Read the model definition and answer for the solid it produces. Units are mm, in the model's axes. Coordinates: 2 decimals unless noted, no trailing zeros. Order: outer loops, then holes, each group sorted by start corner. A loop starts at its lowest first (then second) coordinate and runs counter-clockwise, first axis right, second up. Notation, with made-up numbers: (15, -32.75) - (64, -32.75) arc R15 ccw to (64, -25.75) - close; hole circle Ø7 at (85.25, 60.5). An arc over 180 degrees is marked (long way). Use one line per item in the form item = value.
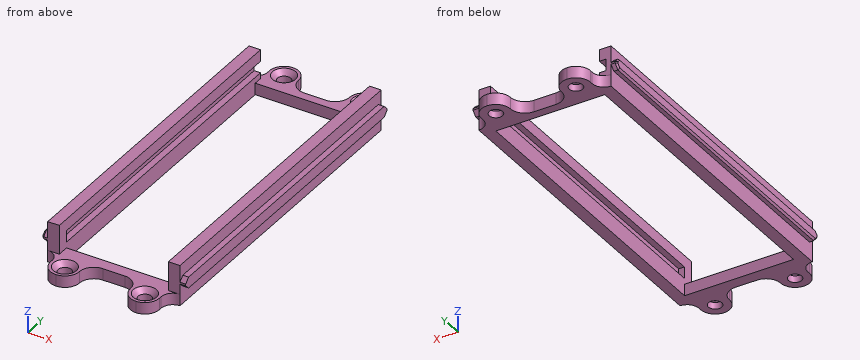
Autodesk Fusion 360 part; units mm, degrees
sketch "Sketch1" plane through (0, 0, 0) normal (1, 0, 0) x (0, 1, 0)
  line L0 (0, 0) -> (56.1898, 0)
  line L1 (56.1898, 0) -> (56.1898, 7)
  line L2 (56.1898, 7) -> (0, 7)
  line L3 (0, 7) -> (0, 0)
  dimension "d1" = 7
extrude "Extrude1" add sketch "Sketch1" along normal blind 1
sketch "Sketch2" plane through (1, 0, 0) normal (1, 0, 0) x (0, 1, 0)
  line L0 (0, 7) -> (0, 0)
  line L1 (0, 0) -> (56.1898, 0)
  line L2 (56.1898, 0) -> (56.1898, 7)
  line L3 (56.1898, 7) -> (0, 7)
  line L4 (0, 0) -> (56.1898, 0)
  line L5 (56.1898, 0) -> (56.1898, 3)
  line L6 (56.1898, 3) -> (0, 3)
  line L7 (0, 3) -> (0, 0)
  line L8 (0, 7) -> (56.1898, 7)
  line L9 (56.1898, 7) -> (56.1898, 5)
  line L10 (56.1898, 5) -> (0, 5)
  line L11 (0, 5) -> (0, 7)
  line L12 (0, 3) -> (2, 3)
  line L13 (2, 3) -> (2, 5)
  line L14 (2, 5) -> (0, 5)
  line L15 (0, 5) -> (0, 3)
  dimension "d4" = 3
  dimension "d5" = 2
  dimension "d12" = 2
extrude "Extrude2" add sketch "Sketch2" along normal blind 1 contours L0 L2 L3 L8 L9 L10 L11 L14 | L0 L6 L10 L12 L13 L14 L15 | L0 L1 L2 L4 L5 L6 L7 L12
sketch "Sketch3" plane through (0, 0, 0) normal (-1, 0, 0) x (0, -1, 0)
  line L0 (0, 0) -> (0, 7)
  line L1 (0, 7) -> (-56.1898, 7)
  line L2 (-56.1898, 7) -> (-56.1898, 0)
  line L3 (-56.1898, 0) -> (0, 0)
  line L4 (-56.1898, 3) -> (0, 3)
  line L5 (0, 3) -> (0, 4.9)
  line L6 (0, 4.9) -> (-56.1898, 4.9)
  line L7 (-56.1898, 4.9) -> (-56.1898, 3)
  dimension "d8" = 1.9
  dimension "d9" = 3
extrude "Extrude3" add sketch "Sketch3" along normal blind 1 contours L0 L2 L4 L5 L6 L7
sketch "Sketch4" plane through (2, 0, 0) normal (1, 0, 0) x (0, 1, 0)
  line L0 (0, 7) -> (0, 0)
  line L1 (0, 0) -> (56.1898, 0)
  line L2 (56.1898, 0) -> (56.1898, 3)
  line L3 (56.1898, 3) -> (2, 3)
  line L4 (2, 3) -> (2, 5)
  line L5 (2, 5) -> (56.1898, 5)
  line L6 (56.1898, 5) -> (56.1898, 7)
  line L7 (56.1898, 7) -> (0, 7)
  line L8 (0, 0) -> (2, 0)
  line L9 (2, 0) -> (2, 2)
  line L10 (2, 2) -> (0, 2)
  line L11 (0, 2) -> (0, 0)
  line L12 (56.1898, 0) -> (54.6898, 0)
  line L13 (54.6898, 0) -> (54.6898, 2)
  line L14 (54.6898, 2) -> (56.1898, 2)
  line L15 (56.1898, 2) -> (56.1898, 0)
  dimension "d13" = 2
  dimension "d14" = 2
  dimension "d15" = 1.5
  dimension "d16" = 2
extrude "Extrude4" add sketch "Sketch4" along normal blind 9.4 contours L0 L1 L8 L9 L10 L11 | L1 L2 L12 L13 L14 L15
mirror "Mirror1" about plane through (11.4, 0, 0) normal (1, 0, 0) of bodies 1 merged
extrude "Extrude5" cut 1 faces at (1, 20.0633, 4.3333) along direction (1, 0, 0) blind 0.1
extrude "Extrude6" cut 1 faces at (1, 20.0633, 4.3333) along direction (-1, 0, 0) blind 0.1
sketch "Sketch5" plane through (0, 0, 0) normal (0, 0, -1) x (1, 0, 0)
  line L0 (20.8, -54.6898) -> (2, -54.6898)
  line L1 (2, -54.6898) -> (2, -2)
  line L2 (2, -2) -> (20.8, -2)
  line L3 (20.8, -2) -> (20.8, -54.6898)
  line L4 (0, -56.1898) -> (22.8, -56.1898)
  line L5 (22.8, -56.1898) -> (22.8, 0)
  line L6 (22.8, 0) -> (0, 0)
  line L7 (0, 0) -> (0, -56.1898)
  line L8 (2, 0) -> (7, 0)
  line L9 (7, 0) -> (7, 5)
  line L10 (7, 5) -> (2, 5)
  line L11 (2, 5) -> (2, 0)
  line L12 (15.8, 0) -> (20.8, 0)
  line L13 (20.8, 0) -> (20.8, 5)
  line L14 (20.8, 5) -> (15.8, 5)
  line L15 (15.8, 5) -> (15.8, 0)
  line L16 (2, -56.1898) -> (7, -56.1898)
  line L17 (7, -56.1898) -> (7, -61.1898)
  line L18 (7, -61.1898) -> (2, -61.1898)
  line L19 (2, -61.1898) -> (2, -56.1898)
  line L20 (15.8, -56.1898) -> (20.8, -56.1898)
  line L21 (20.8, -56.1898) -> (20.8, -61.1898)
  line L22 (20.8, -61.1898) -> (15.8, -61.1898)
  line L23 (15.8, -61.1898) -> (15.8, -56.1898)
  dimension "d25" = 5
  dimension "d26" = 5
  dimension "d27" = 5
  dimension "d28" = 5
  dimension "d30" = 2
  dimension "d31" = 2
  dimension "d32" = 5
  dimension "d33" = 5
  dimension "d34" = 5
  dimension "d35" = 5
  dimension "d36" = 2
  dimension "d37" = 2
extrude "Extrude7" add sketch "Sketch5" against normal blind 2 contours L4 L16 L17 L18 L19 | L6 L8 L9 L10 L11 | L4 L20 L21 L22 L23 | L6 L12 L13 L14 L15
sketch "Sketch6" plane through (0, 0, 2) normal (0, 0, 1) x (-1, 0, 0)
  line L0 (-2, -2) -> (-2, 0)
  line L1 (-2, 0) -> (-2, 5)
  line L2 (-2, 5) -> (-7, 5)
  line L3 (-7, 5) -> (-7, 0)
  line L4 (-7, 0) -> (-15.8, 0)
  line L5 (-15.8, 0) -> (-15.8, 5)
  line L6 (-15.8, 5) -> (-20.8, 5)
  line L7 (-20.8, 5) -> (-20.8, 0)
  line L8 (-20.8, 0) -> (-20.8, -2)
  line L9 (-20.8, -2) -> (-2, -2)
  circle A0 centre (-4.5, 2.5) radius 0.5
  circle A1 centre (-18.3, 2.5) radius 0.5
  circle A2 centre (-4.5, -58.6898) radius 0.5
  circle A3 centre (-18.3, -58.6898) radius 0.5
  line L10 (-7, -61.1898) -> (-2, -61.1898)
  dimension "d40" = 1
  dimension "d41" = 1
  dimension "d42" = 1
  dimension "d43" = 1
  dimension "d44" = 2.5
  dimension "d45" = 2.5
  dimension "d46" = 2.5
  dimension "d47" = 2.5
hole "Hole1" at (4.5, 58.6898, 2) at (18.3, 58.6898, 2) at (4.5, -2.5, 2) at (18.3, -2.5, 2) direction (0, 0, -1) diameter 2.3 depth 17 tip angle 180 countersink diameter 4 countersink angle 90
fillet "Fillet1" radius 2.5 12 edges at (7, -5, 1) (7, 0, 1) (2, -5, 1) (15.8, -5, 1) (20.8, -5, 1) (15.8, 0, 1) (20.8, 61.1898, 1) (15.8, 61.1898, 1) (7, 56.1898, 1) (7, 61.1898, 1) (2, 61.1898, 1) (15.8, 56.1898, 1)
fillet "Fillet1" radius 2 4 edges at (2, 56.1898, 1) (20.8, 56.1898, 1) (20.8, 0, 1) (2, 0, 1)
chamfer "Chamfer1" distance 0.8 angle 45 8 edges at (-0.5, 0, 4.9) (-0.5, 0, 3) (23.3, 0, 3) (23.3, 0, 4.9) (23.3, 56.1898, 4.9) (23.3, 56.1898, 3) (-0.5, 56.1898, 3) (-0.5, 56.1898, 4.9)
chamfer "Chamfer1" distance 0.3 angle 45 2 faces at (-1, 37.4599, 4.2667) (-1, 37.4599, 4.2667)
equation "d17 = ( 20.8 / 2 ) * 1 mm - 1 mm"
(1) Section B-B, the plane y = 39 is taken. Write down the section's boundary in (x, z).
Answer list:
outline = (-1, 3.3) - (-0.7, 3) - (0, 3) - (0, 0) - (2, 0) - (2, 3) - (0.9, 3) - (0.9, 5) - (2, 5) - (2, 7) - (0, 7) - (0, 4.9) - (-0.7, 4.9) - (-1, 4.6) - close; (20.8, 0) - (22.8, 0) - (22.8, 3) - (23.8, 3) - (23.8, 4.9) - (22.8, 4.9) - (22.8, 7) - (20.8, 7) - (20.8, 5) - (21.8, 5) - (21.8, 3) - (20.8, 3) - close
(2) Straight lines are drawn through the part: L1, parallel to Y at x = 4.5, z = 0.65; L2, parallel to X at y = -2.5, z = 0.35; L3, parallel to X at y = 44, z = 3.5. For each, find the intervals that lie inside material, in ascending order.
Answer list:
L1 = -5 to -3.65, -1.35 to 2, 54.69 to 57.54, 59.84 to 61.19
L2 = 2 to 3.35, 5.65 to 7, 15.8 to 17.15, 19.45 to 20.8
L3 = -1 to 0.9, 21.8 to 23.8
(3) Section A-A, the plane x = 11.5 is taken. Write down the section's boundary in (y, z), then the cut area to 3 significant figures.
Answer list:
outline = (0, 0) - (2, 0) - (2, 2) - (0, 2) - close; (54.69, 0) - (56.19, 0) - (56.19, 2) - (54.69, 2) - close
area = 7.00 mm2
(4) Given pin 1 Ø2 at (x, z) = (12, 0.5) entering from +Y; pin 2 Ø1 at (x, z) = (12, 1) entering from -Y; pin 3 Ø2 at (x, z) = (2, 2.5) entering from -Y, each flat-ended and moving along its own axis, determine where each tip first touches the part or whether it passes through.
Answer list:
pin_1 = 56.19
pin_2 = 0
pin_3 = -4.39
